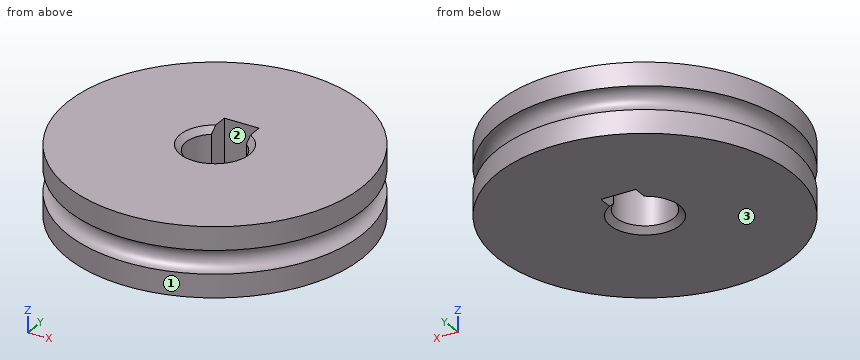
```python
from build123d import *

# Parameters (mm, degrees)
SKETCH_3_R          = 25.45
SKETCH_3_R_2        = 5
EXTRUDE_1_DEPTH     = 12
CHAMFER_1_SIZE      = 1
CUT_EXTRUDE_1_DEPTH = 19
SKETCH_6_R          = 2


with BuildPart() as part:
    # 草图3 → 凸台-拉伸1 (new body)
    with BuildSketch(Plane.XY):
        Circle(SKETCH_3_R)
        Circle(SKETCH_3_R_2, mode=Mode.SUBTRACT)
    extrude(amount=EXTRUDE_1_DEPTH)

    # 倒角1
    chamfer_1_edges = [part.edges().sort_by_distance(p)[0] for p in [
        (-5, 0, 0),
        (-5, 0, 12),
    ]]
    chamfer(chamfer_1_edges, length=CHAMFER_1_SIZE)

    # 草图8 → 切除-拉伸1 (cut)
    with BuildSketch(Plane(origin=(0, 0, 0), x_dir=(-1, 0, 0), z_dir=(0, 0, -1))):
        Polygon((0, 7.65), (-3, 7.65), (-3, 0), (0, 0), (3, 0), (3, 7.65), align=None)
    extrude(amount=-CUT_EXTRUDE_1_DEPTH, mode=Mode.SUBTRACT)

    # 草图6 → 切除-旋转1 (revolve, cut)
    with BuildSketch(Plane(origin=(0, 0, 0), x_dir=(1, 0, 0), z_dir=(0, 1, 0))):
        with Locations((25.45, -6)):
            Circle(SKETCH_6_R)
    revolve(axis=Axis((0, 0, 0), (0, 0, -1)), mode=Mode.SUBTRACT)


solid = part.part
```
The model under review builds one solid part; all positions refer to its coordinate system, in mm. Face numbers are marked on the shaded views. Round coordinates to 2 decimals unless told otherwise and drop trailing zeros. Loops run counter-clockwise (first coordinate to the right, second up) from the corner with the lowest first, then second, coordinate; pieces in that order, holes last.
1) Clearance check with flat-ended pins moving along their axes: P1, Ø1.5, axis at x = 5, z = 2.5, coming from the -Y side; P2, Ø1.5, axis at y = -9, z = 7.5, coming from the -X side; P3, Ø3, axis at y = 6, z = 3.5, coming from the -X side; P4, Ø8, axis at x = 0, y = 0, coming from the +Z side. State where each tip first meets the part, or that it passes through.
Values follow:
P1: stops at y = -25.09
P2: stops at x = -24.01
P3: stops at x = -25.05
P4: passes through
2) Consider section C-C on z = 9.5. State the section outline as (x, y) points, then the cut area to 3 significant figures.
Values follow:
outline: circle Ø50.9 at (0, 0); hole (-3, 4) arc R5 ccw (long way) to (3, 4) - (3, 7.65) - (-3, 7.65) - close
area: 1,940 mm2
3) Wall thickness on line 1 along Y through (x, z) = (0, 3); line 2 along X through (y, z) = (0, 8.5); line 3 along Y through (x, z) = (-2, 8.25): over which ranges is each line inside the solid? List them lowest first.
Values follow:
line 1: y = -25.45 to -5, 7.65 to 25.45
line 2: x = -25.45 to -5, 5 to 25.45
line 3: y = -25.37 to -4.58, 7.65 to 25.37
4) Consider section A-A on x = 0. State the section outline as (y, z) points, then the cut area to 3 significant figures.
Values follow:
outline: (-25.45, 0) - (-6, 0) - (-5, 1) - (-5, 11) - (-6, 12) - (-25.45, 12) - (-25.45, 8) arc R2 cw to (-25.45, 4) - close; (7.65, 0) - (25.45, 0) - (25.45, 4) arc R2 cw to (25.45, 8) - (25.45, 12) - (7.65, 12) - close
area: 445 mm2
5) The part is to be moulded in two halves that separate along X. For the marked faces 1, 2 and 3, say which applies: pulls with the +X half, pulls with the -X half, needs draft (parallel to the pull), parting line crosses it, or undercut.
Values follow:
face 1: parting line crosses it
face 2: undercut
face 3: needs draft
6) Consider section B-B on y = 0. State the section outline as (x, z) points.
Values follow:
outline: (-25.45, 0) - (-6, 0) - (-5, 1) - (-5, 11) - (-6, 12) - (-25.45, 12) - (-25.45, 8) arc R2 cw to (-25.45, 4) - close; (5, 1) - (6, 0) - (25.45, 0) - (25.45, 4) arc R2 cw to (25.45, 8) - (25.45, 12) - (6, 12) - (5, 11) - close
